Geometry: final body of the model. Coordinates: model frame, mm. A direction names the side the tool comes from. Round coordinates to 2 decimals unless told otherwise and drop trailing zeros. Write each loop counter-clockwise with the first axis right and the second up, starting at its lowest first coordinate (ties: lowest second). Pieces come first, ordered by that corner, then holes. Notation, with made-up numbers: (39.25, -10) - (92.25, -10) arc R16 ccw to (92.25, -2) - close; hole circle Ø11 at (9.5, 3.25). An arc over 180 degrees is marked (long way). Write each question's results on one line, items separated by ' | '.
from build123d import *

# Parameters (mm, degrees)
F0_W         = 20
F0_H         = 20
F1_DEPTH     = 3
F3_DEPTH     = 9
F4_R         = 9.99999
F5_T3_DEPTH  = 53
F5_S4_R      = 3
F5_T5_DEPTH  = 29
F5_T8_DEPTH  = 53
F5_S9_R      = 3
F5_T10_DEPTH = 29
F6_R         = 1
F7_DEPTH     = 25
F9_DEPTH     = 3


# Not quite as in the source:
# - a fillet or chamfer that OpenCascade refuses, or shapes differently, is made with other operations: its cross-section is extruded or revolved along the edge and cut away or added
# - a fillet or chamfer is up to 0.001 mm smaller than in the source, because OpenCascade refuses the exact size


with BuildPart() as f1:
    # F0 (on Right) → F1 (new body)
    with BuildSketch(Plane.YZ):
        with Locations((28.7687871605, 25.2807487535)):
            Rectangle(F0_W, F0_H)
    extrude(amount=F1_DEPTH)

    # F2 (on face) → F3 (join)
    with BuildSketch(Plane.XZ.offset(-18.7687871605)):
        with BuildLine():
            Line((3, 22.2807487535), (3, 28.2807487535))
            ThreePointArc((3, 28.2807487535), (0.8786796564, 27.4020690971), (0, 25.2807487535))
            ThreePointArc((0, 25.2807487535), (0.8786796564, 23.15942841), (3, 22.2807487535))
        make_face()
    extrude(amount=F3_DEPTH)

    # F4 (radius 10 in the source; OpenCascade refuses exactly that, so slightly less here)
    f4_edges = [f1.edges().sort_by_distance(p)[0] for p in [
        (1.5, 38.768787, 35.280749),
        (1.5, 38.768787, 15.280749),
    ]]
    fillet(f4_edges, radius=F4_R)

    # F5: fillet of radius 10 on 2 edges, made by hand


with BuildPart() as f5_tool1:
    # F5_s2 → F5_t3 (new body)
    with BuildSketch(Plane.YZ.offset(-25)):
        with BuildLine():
            ThreePointArc((18.7687871605, 25.2807487535), (21.6977193487, 32.3518165654), (28.7687871605, 35.2807487535))
            Line((28.7687871605, 35.2807487535), (18.7687871605, 35.2807487535))
            Line((18.7687871605, 35.2807487535), (18.7687871605, 25.2807487535))
        make_face()
    extrude(amount=F5_T3_DEPTH)

    # F5_s4 → F5_t5 (cut, symmetric)
    with BuildSketch(Plane.XZ.offset(-23.8)):
        with Locations((3, 25.2807487535)):
            Circle(F5_S4_R)
    extrude(amount=F5_T5_DEPTH, both=True, mode=Mode.SUBTRACT)


with BuildPart() as f5_tool6:
    # F5_s7 → F5_t8 (new body)
    with BuildSketch(Plane.YZ.offset(-25)):
        with BuildLine():
            ThreePointArc((28.7687871605, 15.2807487535), (21.6977193487, 18.2096809417), (18.7687871605, 25.2807487535))
            Line((18.7687871605, 25.2807487535), (18.7687871605, 15.2807487535))
            Line((18.7687871605, 15.2807487535), (28.7687871605, 15.2807487535))
        make_face()
    extrude(amount=F5_T8_DEPTH)

    # F5_s9 → F5_t10 (cut, symmetric)
    with BuildSketch(Plane.XZ.offset(-23.8)):
        with Locations((3, 25.2807487535)):
            Circle(F5_S9_R)
    extrude(amount=F5_T10_DEPTH, both=True, mode=Mode.SUBTRACT)


with BuildPart() as f1_1:
    add(f1.part)

    # F5_t11: cut F5_tool1, F5_tool6
    add([f5_tool1.part, f5_tool6.part], mode=Mode.SUBTRACT)

    # F6 (on face) → F7 (cut)
    with BuildSketch(Plane(origin=(0, 0, 0), x_dir=(0, -1, 0), z_dir=(-1, 0, 0))):
        with Locations((-28.7687871605, 25.2807487535)):
            Circle(F6_R)
    extrude(amount=-F7_DEPTH, mode=Mode.SUBTRACT)

    # F8 (on face) → F9 (join)
    with BuildSketch(Plane.XZ.offset(-9.7687871605)):
        with BuildLine():
            Line((3, 28.2807487535), (3, 28.7807487535))
            ThreePointArc((3, 28.7807487535), (-0.5, 25.2807487535), (3, 21.7807487535))
            Line((3, 21.7807487535), (3, 22.2807487535))
            ThreePointArc((3, 22.2807487535), (0, 25.2807487535), (3, 28.2807487535))
        make_face()
        with BuildLine():
            Line((3, 22.2807487535), (3, 28.2807487535))
            ThreePointArc((3, 28.2807487535), (0, 25.2807487535), (3, 22.2807487535))
        make_face()
    extrude(amount=F9_DEPTH)


solid = f1_1.part
Q1. Pin query (flat end, axial travel): pin 1 (6 mm diameter, centred on y = 17, z = 21.5, fed in from -X). Return the tip coordinate at first contact, or that it passes through.
Answer block:
pin 1: x = 0
Q2. Mould query, pull axis Y, two halves, no side actions, for faces 3 (the flat face through (-0.2, 9.769, 25)), 4 (the cylindrical face through (-0.5, 8.29, 25.36)), 5 (the cylindrical face through (1.52, 35.92, 32.27)). Classes: pulls with the +Y half, pulls with the -Y half, needs draft (parallel to the pull), parting line crosses it, or undercut.
Answer block:
face 3: undercut | face 4: needs draft | face 5: pulls with the +Y half
Q3. Section query B-B, the plane y = 9. Return loops of the section in (x, z).
Answer block:
outline: (3, 21.78) - (3, 28.78) arc R3.5 ccw to start
Q4. Access query for faces 1 (the flat face through (0, 29, 23)), 2 (the cylindrical face through (1.52, 35.76, 18.13)). Directions: +Z, -Z, +X, -X, +Y, -Y. A direction counts if a zero-diameter tool reaches every point of the face in a straight line with its end or side. Return the directions, or none.
Answer block:
face 1: +Z, -Z, -X, +Y | face 2: -Z, +X, -X, +Y
Q5. Section query C-C, the plane z = 30.25. Return loops of the section in (x, y).
Answer block:
outline: (0, 20.09) - (3, 20.09) - (3, 37.45) - (0, 37.45) - close
Q6. Ray query, line 1 along Y through (x, z) = (0.3, 25.25); line 2 along X through (y, z) = (37.5, 22); line 3 along Z through (x, y) = (1, 28). Return the intervals inside material, ascending.
Answer block:
line 1: 6.77 to 27.77, 29.77 to 38.77 | line 2: 0 to 3 | line 3: 15.31 to 24.64, 25.92 to 35.25
